Here's how the part is built. I have some questions about the finished solid (model axes, mm). Face numbers are marked on the shaded views. Coordinates: 2 decimals unless noted, no trailing zeros. Loops run counter-clockwise (first coordinate to the right, second up) from the corner with the lowest first, then second, coordinate; pieces in that order, holes last. Notation, with made-up numbers: (22, 0) -> (42, 0) arc R22 cw to (42, 34) -> close; hole circle Ø7 at (44.25, 69). An arc over 180 degrees is marked (long way). Answer as a JSON object with one key per item and string values. Group by question number.
Q1. I want a section at A-A on x = 52.5. Write out the boundary of the cut face in (y, z), then the cut area to 3 significant figures.
Q2. I want a section at D-D on x = -1. Write out the boundary of the cut face in (y, z) (3 decimals).
Q3. I need wall thicknesses on line 1 (X direction, y = 0.4, z = 0); line 2 (Z direction, x = 27.5, y = 2.25); line 3 (Y direction, x = 15, z = 2.5). Which ranges of each line are inside material? Lowest first, please.
Q4. I want a section at C-C on z = 0. Write out the boundary of the cut face in (x, y), then the cut area to 3 significant figures.
Q5. I want a section at B-B on y = 3. Write out the boundary of the cut face in (x, z).
Q6. I'm going to push flat-ended pins straight in: pin 1 (8 mm diameter, centred on x = -3, z = 3, fed in from +Y); pin 2 (0.5 mm diameter, centred on x = 1.5, y = 0.5, fed in from +Z); pin 3 (0.8 mm diameter, centred on x = 2, y = 0.5, fed in from -Z); pin 4 (6 mm diameter, centred on x = -12.5, z = -6.5, fed in from -Y). Where does each tip first touch, or does it pass through?
Q7. Thinking about a two-plate mould opening in Z: for the marked faces 1 and 2, which applies, released by +Z, released by -Z, zero draft, split by the parting line, or undercut?
```python
from build123d import *

# Parameters (mm, degrees)
EXTRUDE_THIN1_DEPTH        = 61.5
EXTRUDE_THIN1_DEPTH_BACK   = 37.5
CUT_EXTRUDE1_REACH         = 66.38
LPATTERN1_COUNT            = 2
LPATTERN1_PITCH            = 25
LPATTERN1_COL_COUNT        = 2
LPATTERN1_COL_PITCH        = 25
SZKIC1_R                   = 1.6
WYTNIJ_WYCI_GNI_CIE1_DEPTH = 65.379732836


with BuildPart() as part:
    # Sketch1 → Extrude-Thin1 (new, two sides: drawn at the far end of the back side and taken through both)
    with BuildSketch(Plane(origin=(0, 0, 0), x_dir=(0, 0, -1), z_dir=(1, 0, 0)).offset(-EXTRUDE_THIN1_DEPTH_BACK)):
        with BuildLine():
            Line((-17.5, 6.5), (-15.5, 6.5))
            ThreePointArc((-15.5, 6.5), (-14.085786438, 5.914213562), (-13.5, 4.5))
            Line((-13.5, 4.5), (-13.5, 2))
            ThreePointArc((-13.5, 2), (-12.914213562, 0.585786438), (-11.5, 0))
            Line((-11.5, 0), (11.5, 0))
            ThreePointArc((11.5, 0), (12.914213562, 0.585786438), (13.5, 2))
            Line((13.5, 2), (13.5, 4.5))
            ThreePointArc((13.5, 4.5), (14.085786438, 5.914213562), (15.5, 6.5))
            Line((15.5, 6.5), (17.5, 6.5))
            Line((17.5, 6.5), (17.5, 7.5))
            Line((17.5, 7.5), (15.5, 7.5))
            ThreePointArc((15.5, 7.5), (13.378679656, 6.621320344), (12.5, 4.5))
            Line((12.5, 4.5), (12.5, 2))
            ThreePointArc((12.5, 2), (12.207106781, 1.292893219), (11.5, 1))
            Line((11.5, 1), (-11.5, 1))
            ThreePointArc((-11.5, 1), (-12.207106781, 1.292893219), (-12.5, 2))
            Line((-12.5, 2), (-12.5, 4.5))
            ThreePointArc((-12.5, 4.5), (-13.378679656, 6.621320344), (-15.5, 7.5))
            Line((-15.5, 7.5), (-17.5, 7.5))
            Line((-17.5, 7.5), (-17.5, 6.5))
        make_face()
    extrude(amount=EXTRUDE_THIN1_DEPTH + EXTRUDE_THIN1_DEPTH_BACK)

    # Sketch2 → Cut-Extrude1 (cut, up to next)
    with BuildSketch(Plane.XZ, mode=Mode.PRIVATE) as cut_extrude1_sk1:
        with BuildLine():
            Line((-5.875, 3.125), (5.875, 3.125))
            ThreePointArc((5.875, 3.125), (9, 0), (5.875, -3.125))
            Line((5.875, -3.125), (-5.875, -3.125))
            ThreePointArc((-5.875, -3.125), (-9, 0), (-5.875, 3.125))
        make_face()
    cut_extrude1_tool1 = extrude(cut_extrude1_sk1.sketch, amount=-CUT_EXTRUDE1_REACH, mode=Mode.PRIVATE) & part.part
    cut_extrude1 = cut_extrude1_tool1.solids().sort_by_distance((0, 0, 0))[0]
    add(cut_extrude1, mode=Mode.SUBTRACT)

    # LPattern1: Cut-Extrude1 ×2
    with Locations(*[(i * LPATTERN1_PITCH, 0, 0) for i in range(1, LPATTERN1_COUNT)]):
        add(cut_extrude1, mode=Mode.SUBTRACT)

    # LPattern1 col: Cut-Extrude1 ×2
    with Locations(*[(-i * LPATTERN1_COL_PITCH, 0, 0) for i in range(1, LPATTERN1_COL_COUNT)]):
        add(cut_extrude1, mode=Mode.SUBTRACT)

    # Szkic1 → Wytnij-wyciągnięcie1 (cut, through all)
    with BuildSketch(Plane.XZ):
        with Locations(Location((52.5, 0, 0), (0, 0, 270))):
            Circle(SZKIC1_R)
    extrude(amount=-WYTNIJ_WYCI_GNI_CIE1_DEPTH, mode=Mode.SUBTRACT)


solid = part.part
```
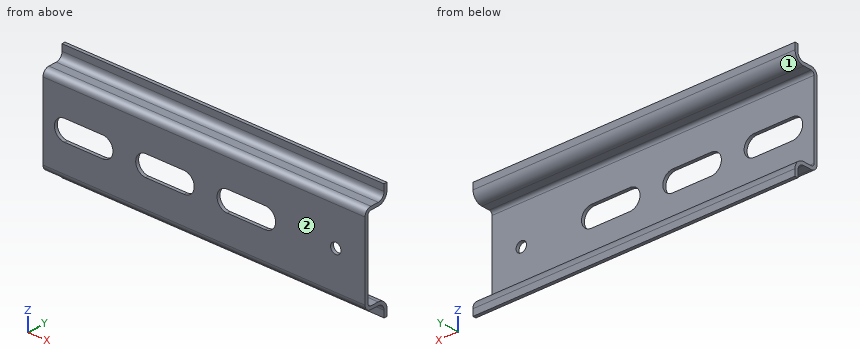
Result set:
{
 "1": {"outline": "(0, -11.5) arc R2 ccw to (2, -13.5) -> (4.5, -13.5) arc R2 cw to (6.5, -15.5) -> (6.5, -17.5) -> (7.5, -17.5) -> (7.5, -15.5) arc R3 ccw to (4.5, -12.5) -> (2, -12.5) arc R1 cw to (1, -11.5) -> (1, -1.6) -> (0, -1.6) -> close; (0, 1.6) -> (1, 1.6) -> (1, 11.5) arc R1 cw to (2, 12.5) -> (4.5, 12.5) arc R3 ccw to (7.5, 15.5) -> (7.5, 17.5) -> (6.5, 17.5) -> (6.5, 15.5) arc R2 cw to (4.5, 13.5) -> (2, 13.5) arc R2 ccw to (0, 11.5) -> close", "area": "41.4 mm²"},
 "2": {"outline": "(0, -11.5) arc R2 ccw to (2, -13.5) -> (4.5, -13.5) arc R2 cw to (6.5, -15.5) -> (6.5, -17.5) -> (7.5, -17.5) -> (7.5, -15.5) arc R3 ccw to (4.5, -12.5) -> (2, -12.5) arc R1 cw to (1, -11.5) -> (1, -3.125) -> (0, -3.125) -> close; (0, 3.125) -> (1, 3.125) -> (1, 11.5) arc R1 cw to (2, 12.5) -> (4.5, 12.5) arc R3 ccw to (7.5, 15.5) -> (7.5, 17.5) -> (6.5, 17.5) -> (6.5, 15.5) arc R2 cw to (4.5, 13.5) -> (2, 13.5) arc R2 ccw to (0, 11.5) -> close"},
 "3": {"line 1": "x = -37.5 to -34, -16 to -9, 9 to 16, 34 to 50.9, 54.1 to 61.5", "line 2": "z = -13.5 to -12.5, 12.5 to 13.5", "line 3": "y = 0 to 1"},
 "4": {"outline": "(-37.5, 0) -> (-34, 0) -> (-34, 1) -> (-37.5, 1) -> close; (-16, 0) -> (-9, 0) -> (-9, 1) -> (-16, 1) -> close; (9, 0) -> (16, 0) -> (16, 1) -> (9, 1) -> close; (34, 0) -> (50.9, 0) -> (50.9, 1) -> (34, 1) -> close; (54.1, 0) -> (61.5, 0) -> (61.5, 1) -> (54.1, 1) -> close", "area": "41.8 mm²"},
 "5": {"outline": "(-37.5, -13.5) -> (61.5, -13.5) -> (61.5, -12.5) -> (-37.5, -12.5) -> close; (-37.5, 12.5) -> (61.5, 12.5) -> (61.5, 13.5) -> (-37.5, 13.5) -> close"},
 "6": {"pin 1": "stops at y = 1", "pin 2": "stops at z = 13.06", "pin 3": "stops at z = -13.17", "pin 4": "stops at y = 0"},
 "7": {"face 1": "undercut", "face 2": "zero draft"}
}
